Geometry check sheet. Reference: drawing and pictorial views, mm from the part's lowest x, y, z. A direction names the side the tool comes from. Coordinates: 2 decimals unless noted, no trailing zeros. Loops run counter-clockwise (first coordinate to the right, second up) from the corner with the lowest first, then second, coordinate; pieces in that order, holes last. Notation, with made-up numbers: (-14.5, 47.25) -> (-2.5, 47.25) arc R23 ccw to (-2.5, 84.25) -> close; hole circle Ø1 at (54, 13). An arc over 180 degrees is marked (long way). Answer as a JSON object with one key per item and string values. Group by question number.
Q1. Set-up check for the marked faces 5 and 6: record each of +Z, -Z, +X, -X, +Y, -Y from which the full face is reachable in a straight line by a thin tool's end or side.
Q2. Cross-section at D-D on z = 2.5. Record the boundary of the cut face in (x, y), and give its area (3 significant figures).
Q3. Cross-section at B-B on z = 16.75. Record the boundary of the cut face in (x, y), and give its area (3 significant figures).
Q4. Gauge pin test, flat ends, axial feed: pin 1 Ø3 at (y, z) = (3, 27) entering from -X; pin 2 Ø2.5 at (x, z) = (35, 31) entering from +Y; pin 3 Ø1.5 at (x, y) = (25.5, 4) entering from -Z; pin 4 Ø1.5 at (y, z) = (9, 28) entering from +X. Record the tip position at first contact, or that the pin passes through.
Q5. Cross-section at A-A on x = 14.5. Record the boundary of the cut face in (y, z), and give its area (3 significant figures).
Q6. Scan lines: L1, parallel to X at y = 2, z = 16.75; L2, parallel to X at y = 6.25, z = 16.75; L3, parallel to Y at x = 22, z = 22. Record each from-to range of solid material in increasing order.
Q7. Cross-section at C-C on y = 2. Give the number of separate pieces and of enclosed holes in the cut face, and give its area (3 significant figures).
Q8. Release check for a two-part mould opening along Z. For the marked faces 1, 2, 3 and 4 record: released by +Z, released by -Z, zero draft, split by the parting line, or undercut.
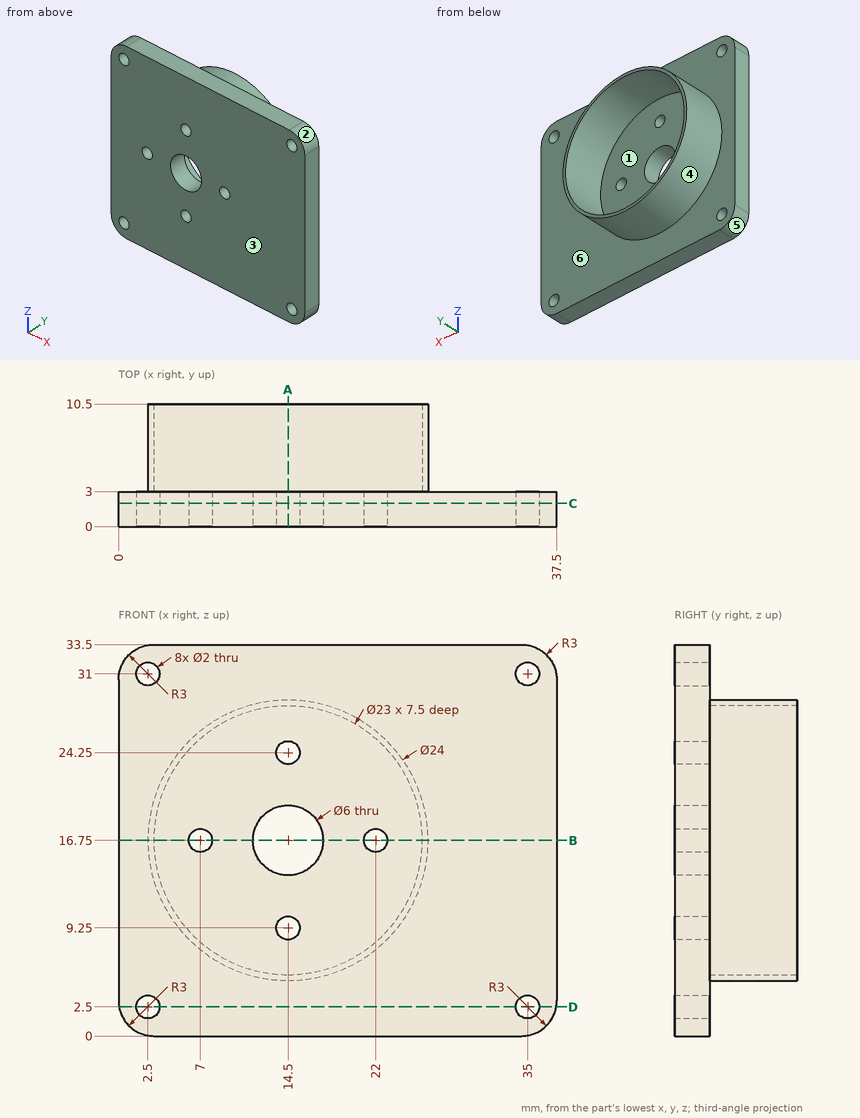
Computed values:
{
 "1": {"face 5": "-Z, -X, +Y, -Y", "face 6": "+Y"},
 "2": {"outline": "(0.04, 0) -> (1.5, 0) -> (1.5, 3) -> (0.04, 3) -> close; (3.5, 0) -> (34, 0) -> (34, 3) -> (3.5, 3) -> close; (36, 0) -> (37.46, 0) -> (37.46, 3) -> (36, 3) -> close", "area": "100 mm²"},
 "3": {"outline": "(0, 0) -> (6, 0) -> (6, 3) -> (3, 3) -> (3, 10.5) -> (2.5, 10.5) -> (2.5, 3) -> (0, 3) -> close; (8, 0) -> (11.5, 0) -> (11.5, 3) -> (8, 3) -> close; (17.5, 0) -> (21, 0) -> (21, 3) -> (17.5, 3) -> close; (23, 0) -> (37.5, 0) -> (37.5, 3) -> (26.5, 3) -> (26.5, 10.5) -> (26, 10.5) -> (26, 3) -> (23, 3) -> close", "area": "90.0 mm²"},
 "4": {"pin 1": "stops at x = 0", "pin 2": "stops at y = 3", "pin 3": "stops at z = 10.51", "pin 4": "stops at x = 20.31"},
 "5": {"outline": "(0, 0) -> (3, 0) -> (3, 4.75) -> (10.5, 4.75) -> (10.5, 5.25) -> (3, 5.25) -> (3, 8.25) -> (0, 8.25) -> close; (0, 10.25) -> (3, 10.25) -> (3, 13.75) -> (0, 13.75) -> close; (0, 19.75) -> (3, 19.75) -> (3, 23.25) -> (0, 23.25) -> close; (0, 25.25) -> (3, 25.25) -> (3, 28.25) -> (10.5, 28.25) -> (10.5, 28.75) -> (3, 28.75) -> (3, 33.5) -> (0, 33.5) -> close", "area": "78.0 mm²"},
 "6": {"L1": "x = 0 to 6, 8 to 11.5, 17.5 to 21, 23 to 37.5", "L2": "x = 2.5 to 3, 26 to 26.5", "L3": "y = 0 to 3"},
 "7": {"separate pieces": "1", "enclosed holes": "9", "area": "1,200 mm²"},
 "8": {"face 1": "undercut", "face 2": "released by +Z", "face 3": "zero draft", "face 4": "split by the parting line"}
}
